from build123d import *

# Parameters (mm, degrees)
SKETCH_W          = 56
SKETCH_H          = 26.5
PAD_DEPTH         = 25
SKETCH001_W       = 51
SKETCH001_H       = 21.5
POCKET_DEPTH      = 0.001
POCKET_DEPTH_BACK = 25.001
SKETCH002_R       = 3.75
POCKET001_DEPTH   = 3.5
SKETCH003_R       = 1.875
POCKET002_DEPTH   = 2.5
CHAMFER_SIZE      = 2.485


with BuildPart() as part:
    # Sketch → Pad (new body)
    with BuildSketch(Plane.XZ):
        Rectangle(SKETCH_W, SKETCH_H)
    extrude(amount=PAD_DEPTH)

    # Sketch001 → Pocket (cut, two sides)
    with BuildSketch(Plane.XZ) as pocket_sk:
        Rectangle(SKETCH001_W, SKETCH001_H)
    extrude(amount=-POCKET_DEPTH, mode=Mode.SUBTRACT)
    extrude(pocket_sk.sketch, amount=POCKET_DEPTH_BACK, mode=Mode.SUBTRACT)

    # Sketch002 (on DatumPlane) → Pocket001 (cut)
    with BuildSketch(Plane(origin=(0, 0, 13.25), x_dir=(-1, 0, 0), z_dir=(0, 0, 1))):
        with Locations((-13.375, 12.5)):
            Circle(SKETCH002_R)
        with Locations((13.375, 12.5)):
            Circle(SKETCH002_R)
    extrude(amount=-POCKET001_DEPTH, mode=Mode.SUBTRACT)

    # Sketch003 (on DatumPlane) → Pocket002 (cut)
    with BuildSketch(Plane(origin=(0, 0, -10.75), x_dir=(-1, 0, 0), z_dir=(0, 0, 1))):
        with Locations((-13.375, 12.5)):
            Circle(SKETCH003_R)
        with Locations((13.375, 12.5)):
            Circle(SKETCH003_R)
    extrude(amount=-POCKET002_DEPTH, mode=Mode.SUBTRACT)

    # Chamfer
    chamfer_edges = [part.edges().sort_by_distance(p)[0] for p in [
        (-11.5, -12.5, -10.75),
        (15.25, -12.5, -10.75),
    ]]
    chamfer(chamfer_edges, length=CHAMFER_SIZE)


solid = part.part
For this review, take the finished solid that the model builds, in its own axes (mm). A direction names the side the tool comes from. Give positions to 0.01 mm unless a question says otherwise; leave off trailing zeros. Loops run counter-clockwise (first coordinate to the right, second up) from the corner with the lowest first, then second, coordinate; pieces in that order, holes last.
Item 1: Draft analysis for pull direction X (two halves, no side actions). For faces 4 (the conical face through (-12.93, -10.52, -13.08)), 5 (the flat face through (-28, -12, 0)), 6 (the flat face through (28, -12, 0)), state which applies: +X half, -X half, draft (parallel to the pull), parting line (faces both ways), or undercut.
Item 2: For line 1 along Z through (x, y) = (-20, -12.75); line 2 along X through (y, z) = (-6.5, -3.5); line 3 along X through (y, z) = (-12.5, -13.2) (3 decimals), list the stretches that pass through material, from the lowest coordinate up.
Item 3: Tool access review of faces 1 (the flat face through (0, -12, -10.75)), 2 (the cylindrical face through (16.139, -15.034, 12.018)), 3 (the conical face through (14.986, -11.265, -13.08)): name each direction out of +Z, -Z, +X, -X, +Y, -Y from which nothing blocks a thin tool from reaching the whole face with its end or side.
Item 4: Take a section at D-D, the plane x = 0.5. State the section outline as (y, z) points, and give its area (3 significant figures).
Item 5: Take a section at A-A, the plane y = -12.5. State the section outline as (x, z) points (3 decimals), and give its area (3 significant figures).
Item 6: Take a section at B-B, the plane z = 1. State the section outline as (x, y) points, and give its area (3 significant figures).
Item 7: Take a section at C-C, the plane y = -17.75. State the section outline as (x, z) points, and give its area (4 significant figures).
Calculated:
1. face 4: undercut
1. face 5: -X half
1. face 6: +X half
2. line 1: z = -13.25 to -10.75, 10.75 to 13.25
2. line 2: x = -28 to -25.5, 25.5 to 28
2. line 3: x = -28 to -15.285, -11.465 to 11.465, 15.285 to 28
3. face 1: +Y, -Y
3. face 2: +Z
3. face 3: none
4. outline: (-25, -13.25) - (0, -13.25) - (0, -10.75) - (-25, -10.75) - close; (-25, 10.75) - (0, 10.75) - (0, 13.25) - (-25, 13.25) - close
4. area: 125 mm2
5. outline: (-28, -13.25) - (-15.25, -13.25) - (-15.25, -13.235) - (-17.735, -10.75) - (-25.5, -10.75) - (-25.5, 10.75) - (-17.125, 10.75) - (-17.125, 13.25) - (-28, 13.25) - close; (-11.5, -13.25) - (11.5, -13.25) - (11.5, -13.235) - (9.015, -10.75) - (-9.015, -10.75) - (-11.5, -13.235) - close; (-9.625, 10.75) - (9.625, 10.75) - (9.625, 13.25) - (-9.625, 13.25) - close; (15.25, -13.25) - (28, -13.25) - (28, 13.25) - (17.125, 13.25) - (17.125, 10.75) - (25.5, 10.75) - (25.5, -10.75) - (17.735, -10.75) - (15.25, -13.235) - close
5. area: 319 mm2
6. outline: (-28, -25) - (-25.5, -25) - (-25.5, 0) - (-28, 0) - close; (25.5, -25) - (28, -25) - (28, 0) - (25.5, 0) - close
6. area: 125 mm2
7. outline: (-28, -13.25) - (28, -13.25) - (28, 13.25) - (-28, 13.25) - close; hole (-25.5, -10.75) - (25.5, -10.75) - (25.5, 10.75) - (-25.5, 10.75) - close
7. area: 387.5 mm2
